For this review, use the dimensioned drawing (mm, ordinates from the lowest corner) and the shaded views. A direction names the side the tool comes from. Give positions to 0.01 mm unless a question says otherwise; leave off trailing zeros. Write each loop counter-clockwise with the first axis right and the second up, starting at its lowest first coordinate (ties: lowest second). Pieces come first, ordered by that corner, then holes. Notation, with made-up numbers: M -30,39 L 2,39 A21 ccw 2,51 Z; hole C 83,-36.5 d11. An arc over 180 degrees is marked long. Use a Markdown table: item, result. Add a question column.
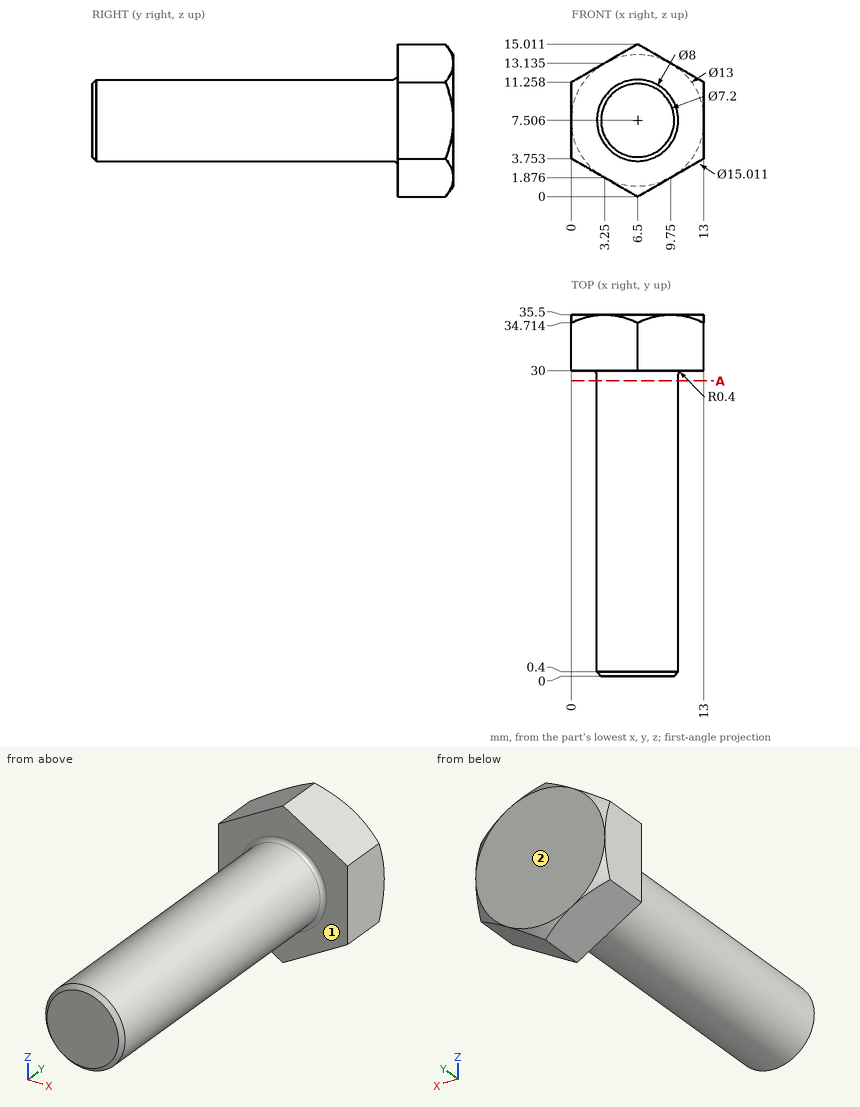
(1) Wall thickness on L1, parallel to Y at x = 10.5, z = 9.75; L2, parallel to X at y = 5, z = 7.25; L3, parallel to Y at x = 2.75, z = 9.25: over which ranges is each line inside the solid? List them lowest first.
(2) Machinability: for the marked faces 1 and 2, which of the approach directions +Z, -Z, +X, -X, +Y, -Y give a long, thin tool a straight path to every point of the face, cutting with its end or side? Answer none if there is none.
(3) For pin 1 (6 mm diameter, centred on y = 24.5, z = 13, fed in from -X); pin 2 (2 mm diameter, centred on y = 6.5, z = 9, fed in from -X); pin 3 (1.5 mm diameter, centred on x = 2, y = 31, fed in from -Z) (1 decimal), all flat-tipped, find the tip position at first contact; note any pin that passes through.
(4) Add section A-A on y = 29. Give the boundary of the cut face in (x, z) (1 decimal).
From the geometry:
| question | item | result |
|---|---|---|
| 1 | L1 | y = 30 to 35.5 |
| 1 | L2 | x = 2.51 to 10.49 |
| 1 | L3 | y = 29.9 to 35.5 |
| 2 | face 1 | -Y |
| 2 | face 2 | +Z, -Z, +X, -X, +Y |
| 3 | pin 1 | stops at x = 3.37 |
| 3 | pin 2 | stops at x = 2.53 |
| 3 | pin 3 | stops at z = 2.2 |
| 4 | outline | C 6.5,7.5 d8 |
